For this review, take the finished solid that the model builds, in its own axes (mm). Give positions to 0.01 mm unless a question says otherwise; leave off trailing zeros. Loops run counter-clockwise (first coordinate to the right, second up) from the corner with the lowest first, then second, coordinate; pieces in that order, holes last. Notation, with made-up numbers: (4, 83) - (25, 83) arc R27 cw to (25, 111) - close; hole circle Ø5 at (19, 47). An arc over 180 degrees is marked (long way). Answer in a Markdown table with one row per item.
```python
from build123d import *

# Parameters (mm, degrees)
SKETCH_W   = 140
SKETCH_H   = 60
SKETCH_R   = 2.5
SKETCH_R_2 = 1
PAD_DEPTH  = 1.8


with BuildPart() as part:
    # Sketch → Pad (new body)
    with BuildSketch(Plane.XY):
        with Locations((68.5, 39.5)):
            Rectangle(SKETCH_W, SKETCH_H)
        with Locations((28.5, 14.5)):
            Circle(SKETCH_R, mode=Mode.SUBTRACT)
        with Locations((108.5, 14.5)):
            Circle(SKETCH_R, mode=Mode.SUBTRACT)
        with Locations((8.5, 24.5)):
            Circle(SKETCH_R, mode=Mode.SUBTRACT)
        with Locations((48.5, 24.5)):
            Circle(SKETCH_R, mode=Mode.SUBTRACT)
        with Locations((88.5, 24.5)):
            Circle(SKETCH_R, mode=Mode.SUBTRACT)
        with Locations((8.5, 44.5)):
            Circle(SKETCH_R, mode=Mode.SUBTRACT)
        with Locations((48.5, 44.5)):
            Circle(SKETCH_R, mode=Mode.SUBTRACT)
        with Locations((88.5, 44.5)):
            Circle(SKETCH_R, mode=Mode.SUBTRACT)
        with Locations((28.5, 54.5)):
            Circle(SKETCH_R, mode=Mode.SUBTRACT)
        with Locations((68.5, 54.5)):
            Circle(SKETCH_R, mode=Mode.SUBTRACT)
        with Locations((108.5, 54.5)):
            Circle(SKETCH_R, mode=Mode.SUBTRACT)
        with Locations((88.5, 64.5)):
            Circle(SKETCH_R, mode=Mode.SUBTRACT)
        with Locations((48.5, 64.5)):
            Circle(SKETCH_R, mode=Mode.SUBTRACT)
        with Locations((8.5, 64.5)):
            Circle(SKETCH_R, mode=Mode.SUBTRACT)
        with Locations((28.5, 34.5)):
            Circle(SKETCH_R, mode=Mode.SUBTRACT)
        with Locations((68.5, 34.5)):
            Circle(SKETCH_R, mode=Mode.SUBTRACT)
        with Locations((108.5, 34.5)):
            Circle(SKETCH_R, mode=Mode.SUBTRACT)
        with Locations((68.5, 14.5)):
            Circle(SKETCH_R, mode=Mode.SUBTRACT)
        with Locations((128.5, 24.5)):
            Circle(SKETCH_R, mode=Mode.SUBTRACT)
        with Locations((128.5, 44.5)):
            Circle(SKETCH_R, mode=Mode.SUBTRACT)
        with Locations((128.5, 64.5)):
            Circle(SKETCH_R, mode=Mode.SUBTRACT)
        with Locations((77.055992, 39.5)):
            Circle(SKETCH_R_2, mode=Mode.SUBTRACT)
        with Locations((122.055992, 39.5)):
            Circle(SKETCH_R_2, mode=Mode.SUBTRACT)
        with Locations((32.055992, 39.5)):
            Circle(SKETCH_R_2, mode=Mode.SUBTRACT)
    extrude(amount=PAD_DEPTH)


solid = part.part
```
1. Mouldability with a two-part tool opening along X and no side actions: class faces 1 (the face through (110.885, 15.251, 0.887)), 2 (the face through (68, 40, 0)) as released by +X, released by -X, zero draft, split by the parting line, or undercut.
Values:
| item | result |
|---|---|
| face 1 | undercut |
| face 2 | zero draft |
2. We need section B-B, the plane x = 88.5. Give the boundary of the cut face in (y, z).
Values:
| item | result |
|---|---|
| outline | (9.5, 0) - (22, 0) - (22, 1.8) - (9.5, 1.8) - close; (27, 0) - (42, 0) - (42, 1.8) - (27, 1.8) - close; (47, 0) - (62, 0) - (62, 1.8) - (47, 1.8) - close; (67, 0) - (69.5, 0) - (69.5, 1.8) - (67, 1.8) - close |
3. Wall thickness on line 1 (Y direction, x = 108.5, z = 1.15); line 2 (Y direction, x = 128.5, z = 1.45); line 3 (X direction, y = 22.5, z = 1.3): over which ranges is each line inside the solid? List them lowest first. Write a range as [from, to].
Values:
| item | result |
|---|---|
| line 1 | y = [9.5, 12], [17, 32], [37, 52], [57, 69.5] |
| line 2 | y = [9.5, 22], [27, 42], [47, 62], [67, 69.5] |
| line 3 | x = [-1.5, 7], [10, 47], [50, 87], [90, 127], [130, 138.5] |
4. We need section A-A, the plane y = 34.5. Give the boundary of the cut face in (x, z), and give its area (3 significant figures).
Values:
| item | result |
|---|---|
| outline | (-1.5, 0) - (26, 0) - (26, 1.8) - (-1.5, 1.8) - close; (31, 0) - (66, 0) - (66, 1.8) - (31, 1.8) - close; (71, 0) - (106, 0) - (106, 1.8) - (71, 1.8) - close; (111, 0) - (138.5, 0) - (138.5, 1.8) - (111, 1.8) - close |
| area | 225 mm^2 |
5. We need section C-C, the plane y = 44.5. Give the boundary of the cut face in (x, z).
Values:
| item | result |
|---|---|
| outline | (-1.5, 0) - (6, 0) - (6, 1.8) - (-1.5, 1.8) - close; (11, 0) - (46, 0) - (46, 1.8) - (11, 1.8) - close; (51, 0) - (86, 0) - (86, 1.8) - (51, 1.8) - close; (91, 0) - (126, 0) - (126, 1.8) - (91, 1.8) - close; (131, 0) - (138.5, 0) - (138.5, 1.8) - (131, 1.8) - close |
6. We need section D-D, the plane z = 1.5. Count the separate pieces of the cut face and the enclosed holes in it, and give its area (3 significant figures).
Values:
| item | result |
|---|---|
| separate pieces | 1 |
| enclosed holes | 24 |
| area | 7,980 mm^2 |
7. Clearance check with a flat-ended pin moving along its axis: pin 1 (4.5 mm diameter, centred on x = 48.5, y = 24.5, fed in from -Z). State where the tip first meets the part, or that it passes through.
Values:
| item | result |
|---|---|
| pin 1 | passes through |
